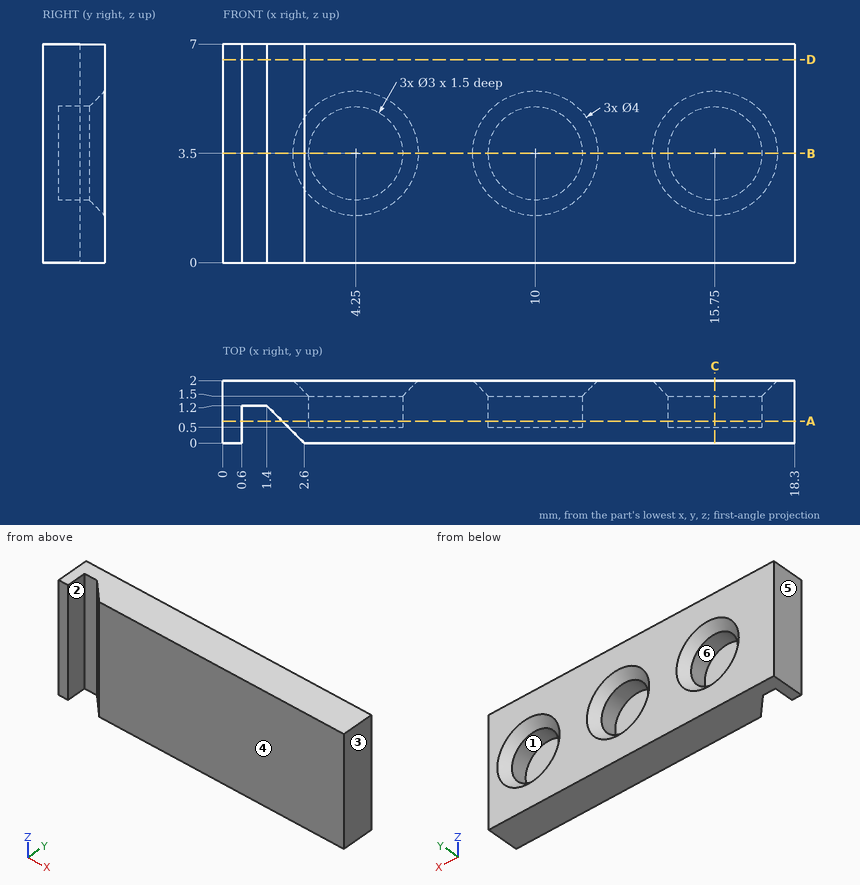
Verification items for this drawing (mm, ordinates from the low corner). A direction names the side the tool comes from. Coordinates: 2 decimals unless noted, no trailing zeros. Write each loop counter-clockwise with the first axis right and the second up, starting at its lowest first coordinate (ties: lowest second). Pieces come first, ordered by that corner, then holes. Notation, with made-up numbers: (-29.5, 77) -> (-17.5, 77) arc R21 cw to (-17.5, 107) -> close; hole circle Ø3 at (24, -16). An arc over 180 degrees is marked (long way). One line per item, written item: value. Start each with the question number.
Q1. Cross-section at D-D on z = 6.5. Enter the section's corners in (x, y).
Q2. Cross-section at C-C on x = 15.75. Enter the section's corners in (y, z), and give its area (3 significant figures).
Q3. Cross-section at B-B on z = 3.5. Enter the section's corners in (x, y).
Q4. Go/stop test with flat-tipped pins: P1, Ø0.9, axis at x = 15.5, z = 4, coming from the +Y side; P2, Ø3.5, axis at x = 10, z = 3.5, coming from the +Y side. Record where each tip stops, or that it passes through.
Q5. Cross-section at A-A on y = 0.7. Enter the section's corners in (x, z), and give its area (3 significant figures).
Q6. Access from +Z, -Z, +X, -X, +Y, -Y to the whole of each face (thin tool, end or side, straight path). Record for the marked faces 1, 2 and 3.
Q7. Mould release check, pull along X, two halves, no side actions. Record for the marked faces 4, 5 and 6: pulls with the +X half, pulls with the -X half, needs draft (parallel to the pull), parting line crosses it, or undercut.
Q8. Thickness scan on L1, parallel to Z at x = 4.25, y = 0.9; L2, parallel to X at y = 1.1, z = 0.75; L3, parallel to Y at x = 3.5, z = 4.5. Record the ranges inside material, lowest first. Write a range as from..to.
Checked values:
1. outline: (0, 0) -> (0.6, 0) -> (0.6, 1.2) -> (1.4, 1.2) -> (2.6, 0) -> (18.3, 0) -> (18.3, 2) -> (0, 2) -> close
2. outline: (0, 0) -> (2, 0) -> (2, 1.5) -> (1.5, 2) -> (0.5, 2) -> (0.5, 5) -> (1.5, 5) -> (2, 5.5) -> (2, 7) -> (0, 7) -> close
2. area: 9.25 mm²
3. outline: (0, 0) -> (0.6, 0) -> (0.6, 1.2) -> (1.4, 1.2) -> (2.6, 0) -> (18.3, 0) -> (18.3, 2) -> (17.75, 2) -> (17.25, 1.5) -> (17.25, 0.5) -> (14.25, 0.5) -> (14.25, 1.5) -> (13.75, 2) -> (12, 2) -> (11.5, 1.5) -> (11.5, 0.5) -> (8.5, 0.5) -> (8.5, 1.5) -> (8, 2) -> (6.25, 2) -> (5.75, 1.5) -> (5.75, 0.5) -> (2.75, 0.5) -> (2.75, 1.5) -> (2.25, 2) -> (0, 2) -> close
4. P1: stops at y = 0.5
4. P2: stops at y = 1.75
5. outline: (0, 0) -> (0.6, 0) -> (0.6, 7) -> (0, 7) -> close; (1.9, 0) -> (18.3, 0) -> (18.3, 7) -> (1.9, 7) -> close; hole circle Ø3 at (4.25, 3.5); hole circle Ø3 at (10, 3.5); hole circle Ø3 at (15.75, 3.5)
5. area: 97.8 mm²
6. face 1: +Y
6. face 2: +Z, -Z, -Y
6. face 3: +Z, -Z, +X, +Y, -Y
7. face 4: needs draft
7. face 5: pulls with the -X half
7. face 6: undercut
8. L1: z = 0..2, 5..7
8. L2: x = 0..0.6, 1.5..18.3
8. L3: y = 0..0.5
